```python
from build123d import *

# Parameters (mm, degrees)
SKETCH1_W                       = 32
SKETCH1_H                       = 21
BOSS_EXTRUDE1_DEPTH             = 8
FILLET1_RADIUS                  = 4
FILLET1_LENGTH                  = 21
CUT_EXTRUDE1_REACH              = 22.742
M2_5_CLEARANCE_HOLE1_AT_2_COUNT = 2
M2_5_CLEARANCE_HOLE1_AT_2_PITCH = 9
FILLET2_R                       = 1
CUT_EXTRUDE2_REACH              = 22.742


with BuildPart() as part:
    # Sketch1 → Boss-Extrude1 (new body)
    with BuildSketch(Plane.XY):
        Rectangle(SKETCH1_W, SKETCH1_H)
    extrude(amount=BOSS_EXTRUDE1_DEPTH)

    # Fillet1: full round fillet: the end face becomes a half cylinder, R = half its width
    fillet1_face = Plane((-16, 0, 4), x_dir=(0, 1, 0), z_dir=(-1, 0, 0))  # on the end face: x along it, z out of the body
    fillet1_slab = fillet1_face.offset(-FILLET1_RADIUS / 2) * Box(FILLET1_LENGTH, 2 * FILLET1_RADIUS, FILLET1_RADIUS, mode=Mode.PRIVATE)  # the body's end, R deep
    fillet1_round = Plane((-12, 0, 4), x_dir=(-1, 0, 0), z_dir=(0, 1, 0)) * Cylinder(FILLET1_RADIUS, FILLET1_LENGTH, mode=Mode.PRIVATE)  # its axis R under the face
    add(fillet1_slab - fillet1_round, mode=Mode.SUBTRACT)

    # Sketch2 → Cut-Extrude1 (cut, up to next)
    with BuildSketch(Plane.XY.offset(8), mode=Mode.PRIVATE) as cut_extrude1_sk1:
        with BuildLine():
            Line((16, 6), (10.291502622, 6))
            ThreePointArc((10.291502622, 6), (-3, 0), (10.291502622, -6))
            Line((10.291502622, -6), (16, -6))
            Line((16, -6), (16, 6))
        make_face()
    cut_extrude1_tool1 = extrude(cut_extrude1_sk1.sketch, amount=-CUT_EXTRUDE1_REACH, mode=Mode.PRIVATE) & part.part
    add(cut_extrude1_tool1.solids().sort_by_distance((6.675863, 0, 8))[0], mode=Mode.SUBTRACT)

    # Sketch5 → M2.5 Clearance Hole1 (revolve, cut)
    with BuildSketch(Plane(origin=(-12, 10.5, 4), x_dir=(0, 0, 1), z_dir=(1, 0, 0))):
        Polygon((0, 0), (0, 4.871247898), (1.45, 4), (1.45, 0), align=None)
    m2_5_clearance_hole1 = revolve(axis=Axis((-12, 16.85, 4), (0, -1, 0)), mode=Mode.SUBTRACT)

    # M2.5 Clearance Hole1 at 2: M2.5 Clearance Hole1 ×2
    with Locations(*[(i * M2_5_CLEARANCE_HOLE1_AT_2_PITCH, 0, 0) for i in range(1, M2_5_CLEARANCE_HOLE1_AT_2_COUNT)]):
        add(m2_5_clearance_hole1, mode=Mode.SUBTRACT)

    # Fillet2
    fillet2_edges = [part.edges().sort_by_distance(p)[0] for p in [
        (16, -8.25, 8),
        (2, 10.5, 8),
        (2, -10.5, 8),
        (2, -10.5, 0),
        (-16, 10.5, 4),
        (-16, -10.5, 4),
        (16, 8.25, 0),
        (16, 8.25, 8),
        (16, 6, 4),
        (16, -6, 4),
        (2, 10.5, 0),
        (16, -8.25, 0),
        (16, 10.5, 4),
        (16, -10.5, 4),
    ]]
    fillet(fillet2_edges, radius=FILLET2_R)

    # Mirror1: M2.5 Clearance Hole1 across plane
    add(m2_5_clearance_hole1.mirror(Plane.ZX), mode=Mode.SUBTRACT)

    # Mirror1 copy 1 sketch → Mirror1 copy 1 (revolve, cut)
    with BuildSketch(Plane(origin=(-3, -10.5, 4), x_dir=(0, 0, 1), z_dir=(1, 0, 0))):
        Polygon((0, 0), (0, -4.871247898), (1.45, -4), (1.45, 0), align=None)
    revolve(axis=Axis((-3, -16.85, 4), (0, -1, 0)), mode=Mode.SUBTRACT)

    # Sketch6 → Cut-Extrude2 (cut, up to next)
    with BuildSketch(Plane.XY, mode=Mode.PRIVATE) as cut_extrude2_sk1:
        with BuildLine():
            Line((-12, 4.5), (-16, 4.5))
            Line((-16, 4.5), (-16, -4.5))
            Line((-16, -4.5), (-12, -4.5))
            ThreePointArc((-12, -4.5), (-7.5, 0), (-12, 4.5))
        make_face()
    cut_extrude2_tool1 = extrude(cut_extrude2_sk1.sketch, amount=CUT_EXTRUDE2_REACH, mode=Mode.PRIVATE) & part.part
    add(cut_extrude2_tool1.solids().sort_by_distance((-12.165908, 0, 0))[0], mode=Mode.SUBTRACT)


solid = part.part
```
CAD build for the part. Positions are in the model's coordinates, mm. A direction names the side the tool comes from. Give positions to 0.01 mm unless a question says otherwise; leave off trailing zeros. Write each loop counter-clockwise with the first axis right and the second up, starting at its lowest first coordinate (ties: lowest second). Pieces come first, ordered by that corner, then holes. Notation, with made-up numbers: M 79.25,43 L 89.25,43 A13 ccw 89.25,52 Z; hole C -19.5,32.25 d5. An arc over 180 degrees is marked long. Return JSON: item names as keys, results as strings. Group by question number.
(1) Band-saw the part on D-D (y = -2.75). Give the cut face in (x, z).
(2) Drill centre lines: L1, parallel to X at y = 8.3, z = 4; L2, parallel to Z at x = -3, y = 7.5; L3, parallel to X at y = 7.25, z = 5.25. Where is each one in solid material? Low to high. Write a range as [from, to].
(3) Band-saw the part on A-A (x = 5). Give the cut face in (y, z), and give its area (3 significant figures).
(4) 3-axis set-ups, long thin cutter, end or side, ignore diameter. For faces 5 (the face through (13, -6, 4)), 6 (the face through (-10.584, 8.528, 3.686)), 7 (the face through (-10.584, -8.528, 3.686)): which of +Z, -Z, +X, -X, +Y, -Y reach the whole face in a straight line?
(5) Flat gauge pins, fed straight in: pin 1 Ø1.5 at (y, z) = (-2.5, 3) entering from -X; pin 2 Ø1.5 at (y, z) = (-1.5, 2) entering from -X; pin 3 Ø2.5 at (x, z) = (-3, 4) entering from +Y. Where does each tip first touch, or does it go through?
(6) Band-saw the part on C-C (x = -10). Give the cut face in (y, z).
(7) Mould opens along Y. For faces 1 (the face through (-3.06, 8.53, 2.55)), 2 (the face through (-3.08, -5.78, 4.24)), 3 (the face through (1.689, 10.215, 7.699)), 4 (the face through (-14, 4.5, 4)) say: pulls with the +Y half, pulls with the -Y half, needs draft (parallel to the pull), parting line crosses it, or undercut.
(8) Band-saw the part on B-B (y = 0). Give the cut face in (x, z), and give its area (3 significant figures).
Entries:
{
 "1": {"outline": "M -8.44,0 L -2.51,0 L -2.51,8 L -8.44,8 Z"},
 "2": {"L1": "x = [-16, -13.45], [-10.55, -4.45], [-1.55, 16]", "L2": "z = [0, 2.55], [5.45, 8]", "L3": "x = [-15.8, -12.73], [-11.27, -3.73], [-2.27, 1.62], [8.38, 16]"},
 "3": {"outline": "M -10.5,1 A1 ccw -9.5,0 L -8,0 L -8,8 L -9.5,8 A1 ccw -10.5,7 Z; M 8,0 L 9.5,0 A1 ccw 10.5,1 L 10.5,7 A1 ccw 9.5,8 L 8,8 Z", "area": "39.1 mm^2"},
 "4": {"face 5": "+Z, -Z, +X", "face 6": "+Y", "face 7": "-Y"},
 "5": {"pin 1": "stops at x = -8.89", "pin 2": "stops at x = -8.1", "pin 3": "stops at y = 6.38"},
 "6": {"outline": "M -10.5,1 A1 ccw -9.5,0 L -4.03,0 L -4.03,8 L -9.5,8 A1 ccw -10.5,7 Z; M 4.03,0 L 9.5,0 A1 ccw 10.5,1 L 10.5,7 A1 ccw 9.5,8 L 4.03,8 Z"},
 "7": {"face 1": "needs draft", "face 2": "pulls with the -Y half", "face 3": "pulls with the +Y half", "face 4": "undercut"},
 "8": {"outline": "M -7.5,0 L -3,0 L -3,8 L -7.5,8 Z", "area": "36.0 mm^2"}
}
